from build123d import *

# Parameters (mm, degrees)
SKETCH1_R           = 6.35
SKETCH1_R_2         = 3.175
BOSS_EXTRUDE1_DEPTH = 177.8
SKETCH7_R           = 9.525
SKETCH7_R_2         = 6.35
BOSS_EXTRUDE2_DEPTH = 6.35


with BuildPart() as part:
    # Sketch1 → Boss-Extrude1 (new body)
    with BuildSketch(Plane(origin=(0, 0, 0), x_dir=(1, 0, 0), z_dir=(0, 1, 0))):
        with Locations(Location((0, 0, 0), (0, 0, 270))):
            Circle(SKETCH1_R)
        with Locations(Location((0, 0, 0), (0, 0, 270))):
            Circle(SKETCH1_R_2, mode=Mode.SUBTRACT)
    extrude(amount=BOSS_EXTRUDE1_DEPTH)

    # Sketch6 → Revolve2 (revolve)
    with BuildSketch(Plane(origin=(0, 0, 0), x_dir=(0, 0, -1), z_dir=(1, 0, 0))):
        with BuildLine():
            Line((0, 177.8), (-44.45, 177.8))
            Line((-44.45, 177.8), (-44.45, 188.815970977))
            ThreePointArc((-44.45, 188.815970977), (-43.947356832, 189.827931199), (-42.837301587, 190.038860096))
            ThreePointArc((-42.837301587, 190.038860096), (-21.620089503, 185.629105586), (0, 184.15))
            Line((0, 184.15), (0, 177.8))
        make_face()
    revolve(axis=Axis((0, 184.15, 0), (0, -1, 0)))

    # Sketch7 → Boss-Extrude2 (add)
    with BuildSketch(Plane.XZ):
        with Locations(Location((0, 0, 0), (0, 0, 270))):
            Circle(SKETCH7_R)
        with Locations(Location((0, 0, 0), (0, 0, 270))):
            Circle(SKETCH7_R_2, mode=Mode.SUBTRACT)
    extrude(amount=-BOSS_EXTRUDE2_DEPTH)


solid = part.part
Here's how the part is built. I have some questions about the finished solid (model axes, mm). A direction names the side the tool comes from. Give positions to 0.01 mm unless a question says otherwise; leave off trailing zeros. Order: outer loops, then holes, each group sorted by start corner. A loop starts at its lowest first (then second) coordinate and runs counter-clockwise, first axis right, second up. Notation, with made-up numbers: M 73,-37 L 104,-37 A30 ccw 104,-2 Z; hole C 59.25,45.25 d6. An arc over 180 degrees is marked long. Answer as a JSON object with one key per item and string values. Group by question number.
1) We'd pull the mould along X, two halves only. Please class faces 1 (the cylindrical face through (-3.86, 90.87, -5.04)), 2 (the cylindrical face through (-1.93, 87.66, -2.52)), 3 (the flat face through (0, 0, -4)): pulls with the +X half, pulls with the -X half, needs draft (parallel to the pull), parting line crosses it, or undercut.
2) Suppose I cut it at A-A, the plane z = 0. Write out the boundary of the cut face in (x, y) (3 decimals), plus the area to 3 significant figures.
3) On a 3-axis mill with a long thin cutter (end or side, diameter ignored), from which of +Z, -Z, +X, -X, +Y, -Y can I reach the whole of each face in a straight line? I mean faces 4 (the flat face through (-6.2, 6.35, -2)), 5 (the cylindrical face through (-13.352, 183.385, 42.397)), 6 (the flat face through (0, 177.8, 0)). Say none if no direction works.
4) I'm going to push flat-ended pins straight in: pin 1 Ø4 at (x, y) = (8.5, 161) entering from -Z; pin 2 Ø10 at (x, z) = (-23.5, 33.5) entering from -Y; pin 3 Ø10 at (x, y) = (6, 163.5) entering from -Z. Where does each tip first touch, or does it pass through?
5) Suppose I cut it at B-B, the plane x = 0. Write out the boundary of the cut face in (y, z) (3 decimals).
6) Please list where these lines run through material, in increasing order: L1, parallel to X at y = 61, z = 0 (3 decimals); L2, parallel to Y at x = -8, z = -3; L3, parallel to X at y = 180.5, z = 0.5. Write a range as [from, to].
7) Suppose I cut it at C-C, the plane y = 174. Write out the boundary of the cut face in (x, z) (3 decimals).
Results found:
{
 "1": {"face 1": "parting line crosses it", "face 2": "undercut", "face 3": "needs draft"},
 "2": {"outline": "M -44.45,177.8 L -6.35,177.8 L -6.35,6.35 L -9.525,6.35 L -9.525,0 L -3.175,0 L -3.175,177.8 L 3.175,177.8 L 3.175,0 L 9.525,0 L 9.525,6.35 L 6.35,6.35 L 6.35,177.8 L 44.45,177.8 L 44.45,188.816 A1.27 ccw 42.837,190.039 A158.75 cw -42.837,190.039 A1.27 ccw -44.45,188.816 Z", "area": "1,920 mm²"},
 "3": {"face 4": "none", "face 5": "+Y, -Y", "face 6": "-Y"},
 "4": {"pin 1": "through", "pin 2": "y = 177.8", "pin 3": "z = -6.27"},
 "5": {"outline": "M 0,-9.525 L 6.35,-9.525 L 6.35,-6.35 L 177.8,-6.35 L 177.8,-44.45 L 188.816,-44.45 A1.27 ccw 190.039,-42.837 A158.75 cw 190.039,42.837 A1.27 ccw 188.816,44.45 L 177.8,44.45 L 177.8,6.35 L 6.35,6.35 L 6.35,9.525 L 0,9.525 L 0,3.175 L 177.8,3.175 L 177.8,-3.175 L 0,-3.175 Z"},
 "6": {"L1": "[-6.35, -3.175], [3.175, 6.35]", "L2": "[0, 6.35], [177.8, 184.38]", "L3": "[-44.45, 44.45]"},
 "7": {"outline": "C 0,0 d12.7; hole C 0,0 d6.35"}
}
